Geometry: final body of the model. Coordinates: model frame, mm. A direction names the side the tool comes from. Give positions to 0.01 mm unless a question says otherwise; leave off trailing zeros. Write each loop counter-clockwise with the first axis right and the second up, starting at its lowest first coordinate (ties: lowest second). Pieces come first, ordered by that corner, then holes.
from build123d import *

# Parameters (mm, degrees)
SKETCH2_R           = 15
BOSS_EXTRUDE1_DEPTH = 3
SKETCH3_R           = 12.9
BOSS_EXTRUDE2_DEPTH = 4
SKETCH4_R           = 0.75
CUT_EXTRUDE1_DEPTH  = 23.338307904


with BuildPart() as part:
    # Sketch2 → Boss-Extrude1 (new body)
    with BuildSketch(Plane.XY):
        Circle(SKETCH2_R)
    extrude(amount=BOSS_EXTRUDE1_DEPTH)

    # Sketch3 → Boss-Extrude2 (add)
    with BuildSketch(Plane(origin=(0, 0, 0), x_dir=(-1, 0, 0), z_dir=(0, 0, -1))):
        Circle(SKETCH3_R)
    extrude(amount=BOSS_EXTRUDE2_DEPTH)

    # Sketch4 → Cut-Extrude1 (cut, through all)
    with BuildSketch(Plane.XY.offset(3)):
        with Locations((-4.5, 0)):
            Circle(SKETCH4_R)
        with Locations((-8, 0)):
            Circle(SKETCH4_R)
        with Locations((-11, 0)):
            Circle(SKETCH4_R)
        with Locations((-3.181980515, 3.181980515)):
            Circle(SKETCH4_R)
        with Locations((-5.656854249, 5.656854249)):
            Circle(SKETCH4_R)
        with Locations((-7.778174593, 7.778174593)):
            Circle(SKETCH4_R)
        with Locations((0, 4.5)):
            Circle(SKETCH4_R)
        with Locations((0, 8)):
            Circle(SKETCH4_R)
        with Locations((0, 11)):
            Circle(SKETCH4_R)
        with Locations((3.181980515, 3.181980515)):
            Circle(SKETCH4_R)
        with Locations((5.656854249, 5.656854249)):
            Circle(SKETCH4_R)
        with Locations((7.778174593, 7.778174593)):
            Circle(SKETCH4_R)
        with Locations((4.5, 0)):
            Circle(SKETCH4_R)
        with Locations((8, 0)):
            Circle(SKETCH4_R)
        with Locations((11, 0)):
            Circle(SKETCH4_R)
        with Locations((3.181980515, -3.181980515)):
            Circle(SKETCH4_R)
        with Locations((5.656854249, -5.656854249)):
            Circle(SKETCH4_R)
        with Locations((7.778174593, -7.778174593)):
            Circle(SKETCH4_R)
        with Locations((0, -4.5)):
            Circle(SKETCH4_R)
        with Locations((0, -8)):
            Circle(SKETCH4_R)
        with Locations((0, -11)):
            Circle(SKETCH4_R)
        with Locations((-3.181980515, -3.181980515)):
            Circle(SKETCH4_R)
        with Locations((-5.656854249, -5.656854249)):
            Circle(SKETCH4_R)
        with Locations((-7.778174593, -7.778174593)):
            Circle(SKETCH4_R)
    extrude(amount=-CUT_EXTRUDE1_DEPTH, mode=Mode.SUBTRACT)


solid = part.part
Q1. Pin query (flat end, axial travel): P1, Ø1.5, axis at x = 2, z = 2, coming from the +Y side. Return the tip coordinate at first contact, or that it passes through.
Filled sheet:
P1: stops at y = 14.95
Q2. Section B-B on x = -8. Output: boundary loops of the cut face in (y, z), plus the area to 3 significant figures.
Filled sheet:
outline: (-12.69, 0) - (-10.12, 0) - (-10.12, -4) - (-8.49, -4) - (-8.49, 3) - (-12.69, 3) - close; (-7.06, -4) - (-0.75, -4) - (-0.75, 3) - (-7.06, 3) - close; (0.75, -4) - (7.06, -4) - (7.06, 3) - (0.75, 3) - close; (8.49, -4) - (10.12, -4) - (10.12, 0) - (12.69, 0) - (12.69, 3) - (8.49, 3) - close
area: 127 mm2
Q3. Ray query, line 1 along Y through (x, z) = (-3.5, -3.5); line 2 along Y through (x, z) = (-3.25, 1); line 3 along X through (y, z) = (-7.5, 1.75). Return the intervals inside material, ascending.
Filled sheet:
line 1: y = -12.42 to -3.86, -2.5 to 2.5, 3.86 to 12.42
line 2: y = -14.64 to -3.93, -2.44 to 2.44, 3.93 to 14.64
line 3: x = -12.99 to -8.47, -7.08 to -0.56, 0.56 to 7.08, 8.47 to 12.99
Q4. Section C-C on y = -4.5. Output: boundary loops of the cut face in (x, z), plus the area to 3 significant figures.
Filled sheet:
outline: (-14.31, 0) - (-12.09, 0) - (-12.09, -4) - (-0.75, -4) - (-0.75, 3) - (-14.31, 3) - close; (0.75, -4) - (12.09, -4) - (12.09, 0) - (14.31, 0) - (14.31, 3) - (0.75, 3) - close
area: 172 mm2
Q5. Pull-direction query (Y, two-part tool) for faces 1 (the cylindrical face through (2.796, -12.593, -1.972)), 2 (the cylindrical face through (-0.55, 8.51, -0.45)), 3 (the flat face through (0, 0, -4)); classes: released by +Y, released by -Y, zero draft, split by the parting line, or undercut.
Filled sheet:
face 1: split by the parting line
face 2: undercut
face 3: zero draft
Q6. Section A-A on x = 0. Count the separate pieces of the cut face and the enclosed holes in it, plus the area to 3 significant figures.
Filled sheet:
separate pieces: 7
enclosed holes: 0
area: 130 mm2
Q7. Access query for faces 4 (the flat face through (4.4, 12.3, 0)), 5 (the cylindrical face through (7.23, 8.29, -0.45)). Directions: +Z, -Z, +X, -X, +Y, -Y. A direction counts if a zero-diameter tool reaches every point of the face in a straight line with its end or side. Return the directions, or none.
Filled sheet:
face 4: -Z
face 5: +Z, -Z
